Part print with two shaded views. Sizes in mm from the minimum x, y, z corner. A direction names the side the tool comes from. Coordinates: 2 decimals unless noted, no trailing zeros. Loops run counter-clockwise (first coordinate to the right, second up) from the corner with the lowest first, then second, coordinate; pieces in that order, holes last.
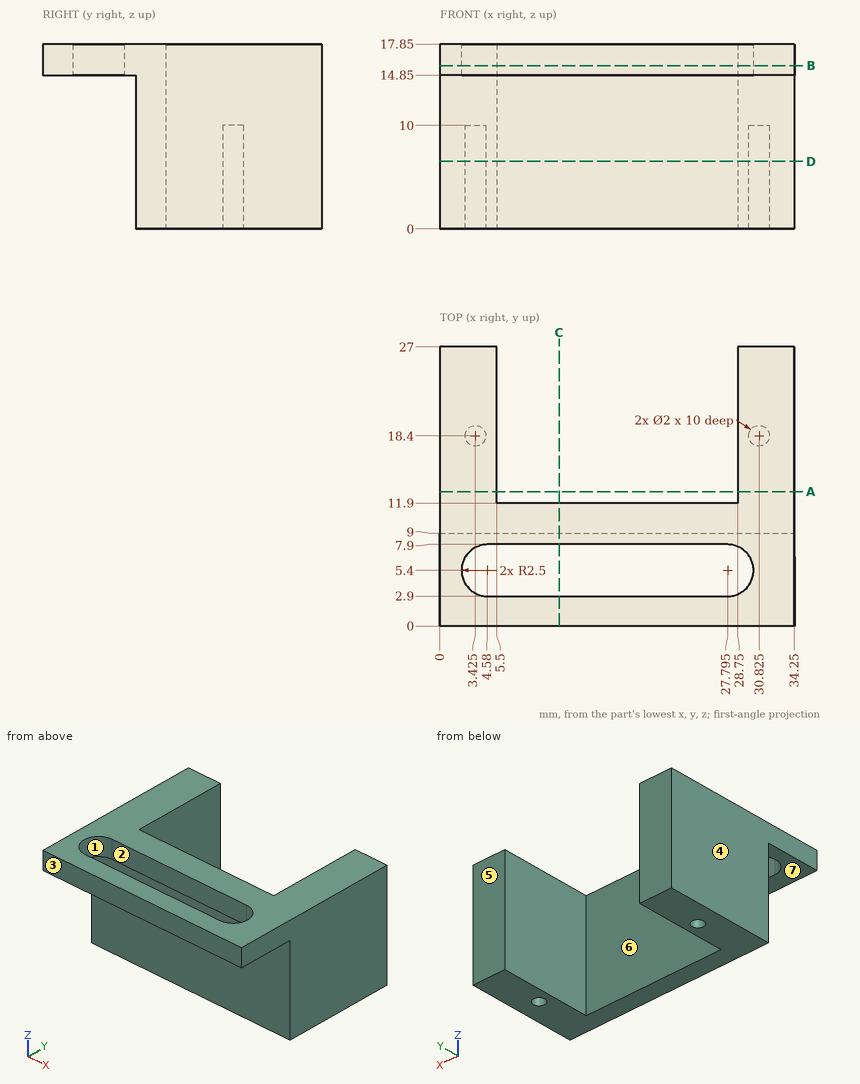
Q1. Slice it at B-B (z = 15.75). List the corners of the cut face in (x, y) (3 decimals).
Answers:
outline: (0, 0) - (34.25, 0) - (34.25, 27) - (28.75, 27) - (28.75, 11.9) - (5.5, 11.9) - (5.5, 27) - (0, 27) - close; hole (4.58, 2.9) - (27.795, 2.9) arc R2.5 ccw to (27.795, 7.9) - (4.58, 7.9) arc R2.5 ccw to start
Q2. Slice it at A-A (y = 13). List the corners of the cut face in (x, z), and give its area (3 significant figures).
Answers:
outline: (0, 0) - (5.5, 0) - (5.5, 17.85) - (0, 17.85) - close; (28.75, 0) - (34.25, 0) - (34.25, 17.85) - (28.75, 17.85) - close
area: 196 mm2
Q3. Slice it at C-C (x = 11.5). List the corners of the cut face in (y, z), and give its area (3 significant figures).
Answers:
outline: (0, 14.85) - (2.9, 14.85) - (2.9, 17.85) - (0, 17.85) - close; (7.9, 14.85) - (9, 14.85) - (9, 0) - (11.9, 0) - (11.9, 17.85) - (7.9, 17.85) - close
area: 63.8 mm2
Q4. Which spindle directions (+Z, -Z, +X, -X, +Y, -Y) get a long thin tool onto all of the face, cutting with end or side? Do the marked faces 5, 6 and 7. Say none if no direction does.
Answers:
face 5: +Z, -Z, +X, -X, +Y
face 6: +Z, -Z, +Y
face 7: -Z, +X, -X, -Y
Q5. Mould opens along Y. For the marked faces 1, 2, 3 and 4 say: +Y half, -Y half, draft (parallel to the pull), parting line (faces both ways), or undercut.
Answers:
face 1: undercut
face 2: undercut
face 3: -Y half
face 4: draft
Q6. Drill centre lines: line 1 (Y direction, x = 26, z = 17.25); line 2 (X direction, y = 15.75, z = 7); line 3 (Y direction, x = 3.5, z = 2.5). Where is each one in solid material? Low to high.
Answers:
line 1: y = 0 to 2.9, 7.9 to 11.9
line 2: x = 0 to 5.5, 28.75 to 34.25
line 3: y = 9 to 17.4, 19.4 to 27
Q7. Flat gauge pins, fed straight in: P1, Ø3, axis at x = 8.5, y = 22, coming from the +Z side; P2, Ø1.5, axis at x = 11, z = 16, coming from the +Y side; P3, Ø7.5, axis at x = 15.5, z = 7.5, coming from the -Y side; P4, Ø2.5, axis at x = 22.5, y = 2.5, coming from the -Z side. Where does each tip first touch, or does it go through?
Answers:
P1: passes through
P2: stops at y = 11.9
P3: stops at y = 9
P4: stops at z = 14.85
Q8. Slice it at D-D (z = 6.5). List the corners of the cut face in (x, y) (3 decimals).
Answers:
outline: (0, 9) - (34.25, 9) - (34.25, 27) - (28.75, 27) - (28.75, 11.9) - (5.5, 11.9) - (5.5, 27) - (0, 27) - close; hole circle Ø2 at (3.425, 18.4); hole circle Ø2 at (30.825, 18.4)
